CAD build for the part. Positions are in the model's coordinates, mm. A direction names the side the tool comes from. Give positions to 0.01 mm unless a question says otherwise; leave off trailing zeros. Loops run counter-clockwise (first coordinate to the right, second up) from the corner with the lowest first, then second, coordinate; pieces in that order, holes last.
Item 1: Saw through at C-C on x = 32.5. Give the cut face in (y, z).
Item 2: Which spindle directions (+Z, -Z, +X, -X, +Y, -Y) get a long thin tool onto all of the face, cutting with end or side? Do faces 1 (the flat face through (0.823, 25.35, 28.347)), 2 (the cylindrical face through (-5.107, 18.773, -12.639)), 3 (the flat face through (-17, 25, 30.319)), 4 (the flat face through (16, 25, 20.319)), 5 (the cylindrical face through (-33.16, 42.35, 3.04)). Say none if no direction does.
Item 3: Probe probe 1 along Z at (x, y) = (20, 33.5); probe 2 along Z at (x, y) = (-8, 8); probe 3 along X at (y, z) = (2, -1). List the from-to ranges inside material, lowest first.
Item 4: Saw through at D-D on z = -6. Give the cut face in (x, y), plus the area to 3 significant figures.
Item 5: Drop flat-ended pins along their axis: P1, Ø7, axis at x = -9.15, y = 17.5, coming from the +Z side; P2, Ø6, axis at x = 55, y = 44.5, coming from the +Z side; P3, Ø3, axis at y = 29, z = -9, coming from the +X side. Give the stop position or say it passes through.
Item 6: Saw through at B-B on y = 29. Give the number of separate pieces and of enclosed holes in the cut face, plus the area to 3 significant figures.
Item 7: Saw through at A-A on x = 14. Give the cut face in (y, z), plus the area to 3 significant figures.
Item 8: Mould opens along X. For faces 6 (the flat face through (-32.149, 17, 13)), 7 (the cylindrical face through (67.657, 24.586, -12.639)), 8 (the flat face through (-9, 18, -15.681)), 9 (the cylindrical face through (22.12, 18.31, -12.64)) say: released by +X, released by -X, zero draft, split by the parting line, or undercut.
from build123d import *

# Parameters (mm, degrees)
SALIENTE_EXTRUIR1_DEPTH = 50
CROQUIS3_R              = 17.5
CORTAR_EXTRUIR1_DEPTH   = 2
CROQUIS4_R              = 10
CORTAR_EXTRUIR2_DEPTH   = 25
CROQUIS5_R              = 11
CORTAR_EXTRUIR3_DEPTH   = 96.884399238
CORTAR_EXTRUIR4_DEPTH   = 96.884399238
CROQUIS7_R              = 2.5
SALIENTE_EXTRUIR6_DEPTH = 4
CORTAR_EXTRUIR6_DEPTH   = 4
CROQUIS10_R             = 4.23710426
CORTAR_EXTRUIR7_DEPTH   = 98.86632729
SALIENTE_EXTRUIR8_DEPTH = 4
CORTAR_EXTRUIR10_DEPTH  = 4


with BuildPart() as part:
    # Croquis2 → Saliente-Extruir1 (new body)
    with BuildSketch(Plane(origin=(0, 0, 0), x_dir=(1, 0, 0), z_dir=(0, 1, 0))):
        with BuildLine():
            Line((-34.14893617, 19.680851064), (-34.14893617, -30.319148936))
            Line((-34.14893617, -30.319148936), (0, -30.319148936))
            Line((0, -30.319148936), (0, -26.319148936))
            Line((0, -26.319148936), (67.659574468, -26.319148936))
            Line((67.659574468, -26.319148936), (67.659574468, -20.319148936))
            Line((67.659574468, -20.319148936), (-17.64893617, -20.319148936))
            ThreePointArc((-17.64893617, -20.319148936), (-18.709596342, -19.879809108), (-19.14893617, -18.819148936))
            Line((-19.14893617, -18.819148936), (-19.14893617, 8.180851064))
            ThreePointArc((-19.14893617, 8.180851064), (-18.709596342, 9.241511236), (-17.64893617, 9.680851064))
            Line((-17.64893617, 9.680851064), (67.659574468, 9.680851064))
            Line((67.659574468, 9.680851064), (67.659574468, 15.680851064))
            Line((67.659574468, 15.680851064), (0, 15.680851064))
            Line((0, 15.680851064), (0, 19.680851064))
            Line((0, 19.680851064), (-34.14893617, 19.680851064))
        make_face()
    extrude(amount=SALIENTE_EXTRUIR1_DEPTH)

    # Croquis3 → Cortar-Extruir1 (cut)
    with BuildSketch(Plane.ZY.offset(34.14893617)):
        with Locations((5.319148936, 25)):
            Circle(CROQUIS3_R)
    extrude(amount=-CORTAR_EXTRUIR1_DEPTH, mode=Mode.SUBTRACT)

    # Croquis4 → Cortar-Extruir2 (cut)
    with BuildSketch(Plane.ZY.offset(32.14893617)):
        with Locations((5.319148936, 25)):
            Circle(CROQUIS4_R)
    extrude(amount=-CORTAR_EXTRUIR2_DEPTH, mode=Mode.SUBTRACT)

    # Croquis5 → Cortar-Extruir3 (cut, through all)
    with BuildSketch(Plane.XY.offset(26.319148936)):
        with Locations((30.85106383, 25)):
            Circle(CROQUIS5_R)
    extrude(amount=-CORTAR_EXTRUIR3_DEPTH, mode=Mode.SUBTRACT)

    # Croquis6 → Cortar-Extruir4 (cut, through all)
    with BuildSketch(Plane.XY.offset(26.319148936)):
        with BuildLine():
            Line((75.592825188, 50), (75.592825188, 0))
            Line((75.592825188, 0), (54.24269842, 0))
            ThreePointArc((54.24269842, 0), (67.659574468, 25), (54.24269842, 50))
            Line((54.24269842, 50), (75.592825188, 50))
        make_face()
    extrude(amount=-CORTAR_EXTRUIR4_DEPTH, mode=Mode.SUBTRACT)

    # Croquis7 → Saliente-Extruir6 (add)
    with BuildSketch(Plane.XY.offset(30.319148936)):
        Polygon((-34.14893617, 50), (-8.14893617, 50), (10.049575543, 0), (-34.14893617, 0), align=None)
        with Locations((-9.14893617, 17.5)):
            Circle(CROQUIS7_R, mode=Mode.SUBTRACT)
    extrude(amount=-SALIENTE_EXTRUIR6_DEPTH)

    # Croquis8 → Cortar-Extruir6 (cut)
    with BuildSketch(Plane.XY.offset(30.319148936)):
        Polygon((0, 27.61098188), (-8.14893617, 50), (0, 50), align=None)
    extrude(amount=-CORTAR_EXTRUIR6_DEPTH, mode=Mode.SUBTRACT)

    # Croquis10 → Cortar-Extruir7 (cut, through all)
    with BuildSketch(Plane.XY.offset(30.319148936)):
        with Locations((-9.14893617, 17.5)):
            Circle(CROQUIS10_R)
    extrude(amount=-CORTAR_EXTRUIR7_DEPTH, mode=Mode.SUBTRACT)

    # Croquis11 → Saliente-Extruir8 (add)
    with BuildSketch(Plane(origin=(0, 0, -19.680851064), x_dir=(-1, 0, 0), z_dir=(0, 0, -1))):
        Polygon((8.14893617, 50), (-10.049575543, 0), (19.14893617, 0), (19.14893617, 50), align=None)
    extrude(amount=-SALIENTE_EXTRUIR8_DEPTH)

    # Croquis13 → Cortar-Extruir10 (cut)
    with BuildSketch(Plane(origin=(0, 0, -19.680851064), x_dir=(-1, 0, 0), z_dir=(0, 0, -1))):
        Polygon((0, 50), (0, 27.61098188), (8.14893617, 50), align=None)
    extrude(amount=-CORTAR_EXTRUIR10_DEPTH, mode=Mode.SUBTRACT)


solid = part.part
Results below:
1. outline: (0, -15.68) - (14.12, -15.68) - (14.12, -9.68) - (0, -9.68) - close; (0, 20.32) - (14.12, 20.32) - (14.12, 26.32) - (0, 26.32) - close; (35.88, -15.68) - (50, -15.68) - (50, -9.68) - (35.88, -9.68) - close; (35.88, 20.32) - (50, 20.32) - (50, 26.32) - (35.88, 26.32) - close
2. face 1: +Z, +X, +Y
2. face 2: +Z
2. face 3: +Z, +X, -X, +Y, -Y
2. face 4: +X, +Y, -Y
2. face 5: -X
3. probe 1: z = -15.68 to -9.68, 20.32 to 26.32
3. probe 2: z = -19.68 to -9.68, 20.32 to 30.32
3. probe 3: x = -34.15 to -19.15
4. outline: (-34.15, 0) - (-19.15, 0) - (-19.15, 50) - (-34.15, 50) - (-34.15, 38.35) - (-32.15, 38.35) - (-32.15, 11.65) - (-34.15, 11.65) - close
4. area: 697 mm2
5. P1: stops at z = -15.68
5. P2: stops at z = 26.32
5. P3: stops at x = 67.54
6. separate pieces: 4
6. enclosed holes: 0
6. area: 1,390 mm2
7. outline: (0, -15.68) - (50, -15.68) - (50, -9.68) - (0, -9.68) - close; (0, 20.32) - (50, 20.32) - (50, 26.32) - (0, 26.32) - close
7. area: 600 mm2
8. face 6: released by -X
8. face 7: released by +X
8. face 8: undercut
8. face 9: undercut
